Geometry: final body of the model. Coordinates: model frame, mm. A direction names the side the tool comes from. Give positions to 0.01 mm unless a question says otherwise; leave off trailing zeros. Loops run counter-clockwise (first coordinate to the right, second up) from the corner with the lowest first, then second, coordinate; pieces in that order, holes last. Notation, with made-up numbers: M 54.25,86 L 71.25,86 A8 cw 71.25,96 Z; hole C 5.5,-19.75 d8. An arc over 180 degrees is marked long. Put each result on its own line as item: value.
```python
from build123d import *

# Parameters (mm, degrees)
F0_W     = 238.125
F0_H     = 168.275
F1_DEPTH = 6.35
F3_DEPTH = 25.4
F4_R     = 5.08
F6_DEPTH = 6.351


with BuildPart() as f1:
    # F0 (on Top) → F1 (new body)
    with BuildSketch(Plane.XY):
        Rectangle(F0_W, F0_H)
    extrude(amount=F1_DEPTH)

    # F2 (on face) → F3 (cut)
    with BuildSketch(Plane.XY.offset(6.35)):
        Polygon((-42.458184, 31.839972), (-55.5625, 44.958), (-55.5625, 0), (-55.5625, -44.958), (-42.458184, -31.839972), (-10.651458, -63.613451), (52.8955, 0), (-10.651458, 63.613451), align=None)
    extrude(amount=-F3_DEPTH, mode=Mode.SUBTRACT)

    # F4
    f4_edges = [f1.edges().sort_by_distance(p)[0] for p in [
        (119.0625, -84.1375, 3.175),
        (119.0625, 84.1375, 3.175),
        (-119.0625, -84.1375, 3.175),
        (-119.0625, 84.1375, 3.175),
    ]]
    fillet(f4_edges, radius=F4_R)

    # F5 (on face) → F6 (cut, through all)
    with BuildSketch(Plane.XY.offset(6.35)):
        with BuildLine():
            Line((-43.013729, 34.19309), (-55.488033, 46.680446))
            ThreePointArc((-55.488033, 46.680446), (-56.346235, 46.851503), (-56.8325, 46.123962))
            Line((-56.8325, 46.123962), (-56.8325, -46.123962))
            ThreePointArc((-56.8325, -46.123962), (-56.346235, -46.851503), (-55.488033, -46.680446))
            Line((-55.488033, -46.680446), (-43.013729, -34.19309))
            ThreePointArc((-43.013729, -34.19309), (-42.457074, -33.962175), (-41.900178, -34.192508))
            Line((-41.900178, -34.192508), (-11.207586, -64.853017))
            ThreePointArc((-11.207586, -64.853017), (-10.65069, -65.08335), (-10.094034, -64.852435))
            Line((-10.094034, -64.852435), (54.13471, -0.556485))
            ThreePointArc((54.13471, -0.556485), (54.365043, 0), (54.13471, 0.556485))
            Line((54.13471, 0.556485), (-10.094034, 64.852435))
            ThreePointArc((-10.094034, 64.852435), (-10.65069, 65.08335), (-11.207586, 64.853017))
            Line((-11.207586, 64.853017), (-41.900178, 34.192508))
            ThreePointArc((-41.900178, 34.192508), (-42.457074, 33.962175), (-43.013729, 34.19309))
        make_face()
    extrude(amount=-F6_DEPTH, mode=Mode.SUBTRACT)


solid = f1.part
```
Item 1: Set-up query: faces 1 (the flat face through (-2, 84.138, 3)), 2 (the flat face through (21.571, -33.155, 3.219)). Return all of +Z, -Z, +X, -X, +Y, -Y with unobstructed straight access to the full face (end or side cutting, diameter ignored); none if empty.
Output values:
face 1: +Z, -Z, +X, -X, +Y
face 2: +Z, -Z
Item 2: Section A-A on z = 1.25. Output: boundary loops of the cut face in (x, y).
Output values:
outline: M -119.06,-79.06 A5.08 ccw -113.98,-84.14 L 113.98,-84.14 A5.08 ccw 119.06,-79.06 L 119.06,79.06 A5.08 ccw 113.98,84.14 L -113.98,84.14 A5.08 ccw -119.06,79.06 Z; hole M -56.83,-46.12 A0.79 ccw -55.49,-46.68 L -43.01,-34.19 A0.79 cw -41.9,-34.19 L -11.21,-64.85 A0.79 ccw -10.09,-64.85 L 54.13,-0.56 A0.79 ccw 54.13,0.56 L -10.09,64.85 A0.79 ccw -11.21,64.85 L -41.9,34.19 A0.79 cw -43.01,34.19 L -55.49,46.68 A0.79 ccw -56.83,46.12 Z
Item 3: Section B-B on x = 5. Output: boundary loops of the cut face in (y, z), then the cut area to 3 significant figures.
Output values:
outline: M -84.14,0 L -49.74,0 L -49.74,6.35 L -84.14,6.35 Z; M 49.74,0 L 84.14,0 L 84.14,6.35 L 49.74,6.35 Z
area: 437 mm²
Item 4: Line query: probe 1 along Y at (x, z) = (-1, 4.75); probe 2 along X at (y, z) = (47, 1.75); probe 3 along X at (y, z) = (-7.5, 3). Output: solid intervals per line, ascending. Write a range as [from, to].
Output values:
probe 1: [-84.14, -55.75], [55.75, 84.14]
probe 2: [-119.06, -29.08], [7.74, 119.06]
probe 3: [-119.06, -56.83], [47.2, 119.06]
Item 5: Mould query, pull axis Y, two halves, no side actions, for faces 3 (the flat face through (119.062, -1, 3)), 4 (the cylindrical face through (-117.614, -82.61, 3.219)), 5 (the flat face through (-56.832, 1, 3)), 6 (the flat face through (-26.769, -49.308, 3.219)). Classes: pulls with the +Y half, pulls with the -Y half, needs draft (parallel to the pull), parting line crosses it, or undercut.
Output values:
face 3: needs draft
face 4: pulls with the -Y half
face 5: undercut
face 6: undercut
Item 6: Section C-C on y = -11. Output: boundary loops of the cut face in (x, z).
Output values:
outline: M -119.06,0 L -56.83,0 L -56.83,6.35 L -119.06,6.35 Z; M 43.7,0 L 119.06,0 L 119.06,6.35 L 43.7,6.35 Z
